Geometry check sheet. Reference: the model listing, model coordinates, mm. Coordinates: 2 decimals unless noted, no trailing zeros. Order: outer loops, then holes, each group sorted by start corner. A loop starts at its lowest first (then second) coordinate and runs counter-clockwise, first axis right, second up. Notation, with made-up numbers: (-34.75, 63) - (-20.75, 63) arc R31 ccw to (-20.75, 96) - close; hole circle Ø7 at (-2, 40). An arc over 180 degrees is marked (long way). Use CSV: the item, a comma, the result in double quotes. Start each with the question number.
1) Sectioned sample at A-A, the plane x = 106.5. Record the cut outline in (y, z), and give its area (3 significant figures).
2) Depth check by flat-ended pin: P1, Ø5, axis at x = 450, z = 0, coming from the +Y side; P2, Ø3.5, axis at x = 153.5, y = 9, coming from the -Z side. Enter the tip coordinate at first touch or a pass-through.
3) Thickness scan on probe 1 along Z at (x, y) = (210, 12.35); probe 2 along Z at (x, y) = (570, 5.75); probe 3 along Z at (x, y) = (63.5, 6.5). Record the ranges inside material, lowest first. Write a range as [from, to].
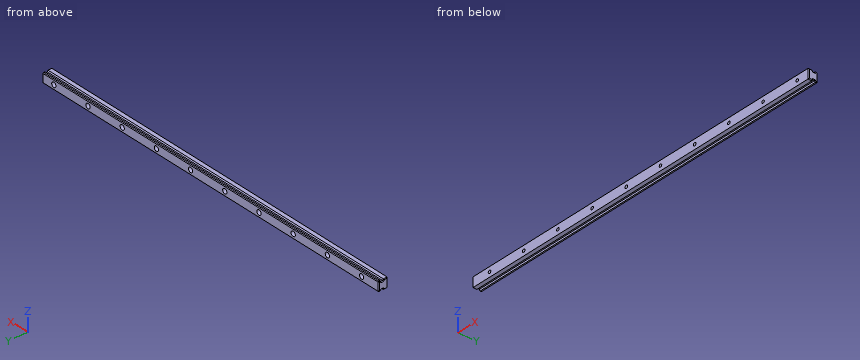
from build123d import *

# Parameters (mm, degrees)
BOSS_EXTRUDE1_DEPTH = 590
CHAMFER1_SIZE       = 1
CHAMFER2_SIZE       = 1
SKETCH2_R           = 3.75
CUT_EXTRUDE1_DEPTH  = 5.3
SKETCH3_R           = 2.25
CUT_EXTRUDE2_DEPTH  = 591.111802966
LPATTERN1_COUNT     = 67
LPATTERN1_PITCH     = 60


with BuildPart() as part:
    # Sketch1 → Boss-Extrude1 (new body)
    with BuildSketch(Plane(origin=(0, 0, 0), x_dir=(0, 0, -1), z_dir=(1, 0, 0))):
        Polygon((-7.5, 0), (7.5, 0), (7.5, 6), (5.5, 7), (5.5, 10), (7.5, 11), (7.5, 13), (6.5, 14), (-6.5, 14), (-7.5, 13), (-7.5, 11), (-5.5, 10), (-5.5, 7), (-7.5, 6), align=None)
    extrude(amount=BOSS_EXTRUDE1_DEPTH)

    # Chamfer1
    chamfer1_edges = [part.edges().sort_by_distance(p)[0] for p in [
        (0, 6.5, 6.5),
        (0, 8.5, 5.5),
        (0, 10.5, 6.5),
        (0, 12, 7.5),
        (0, 13.5, 7),
        (0, 14, 0),
        (0, 13.5, -7),
        (0, 12, -7.5),
        (0, 10.5, -6.5),
        (0, 8.5, -5.5),
        (0, 6.5, -6.5),
        (0, 3, -7.5),
        (0, 0, 0),
        (0, 3, 7.5),
    ]]
    chamfer(chamfer1_edges, length=CHAMFER1_SIZE)

    # Chamfer2
    chamfer2_edges = [part.edges().sort_by_distance(p)[0] for p in [
        (590, 3, -7.5),
        (590, 6.5, -6.5),
        (590, 8.5, -5.5),
        (590, 10.5, -6.5),
        (590, 12, -7.5),
        (590, 13.5, -7),
        (590, 14, 0),
        (590, 13.5, 7),
        (590, 12, 7.5),
        (590, 10.5, 6.5),
        (590, 3, 7.5),
        (590, 8.5, 5.5),
        (590, 6.5, 6.5),
        (590, 0, 0),
    ]]
    chamfer(chamfer2_edges, length=CHAMFER2_SIZE)

    # Sketch2 → Cut-Extrude1 (cut)
    with BuildSketch(Plane(origin=(0, 14, 0), x_dir=(1, 0, 0), z_dir=(0, 1, 0))):
        with Locations(Location((570, 0, 0), (0, 0, 270))):
            Circle(SKETCH2_R)
    cut_extrude1 = extrude(amount=-CUT_EXTRUDE1_DEPTH, mode=Mode.SUBTRACT)

    # Sketch3 → Cut-Extrude2 (cut, through all)
    with BuildSketch(Plane(origin=(0, 8.7, 0), x_dir=(1, 0, 0), z_dir=(0, 1, 0))):
        with Locations(Location((570, 0, 0), (0, 0, 270))):
            Circle(SKETCH3_R)
    cut_extrude2 = extrude(amount=-CUT_EXTRUDE2_DEPTH, mode=Mode.SUBTRACT)

    # LPattern1: Cut-Extrude1, Cut-Extrude2 ×67
    with Locations(*[(-i * LPATTERN1_PITCH, 0, 0) for i in range(1, LPATTERN1_COUNT)]):
        add(cut_extrude1, mode=Mode.SUBTRACT)
        add(cut_extrude2, mode=Mode.SUBTRACT)


solid = part.part
Evaluation:
1,outline,"(0, -7.5) - (6, -7.5) - (7, -5.5) - (10, -5.5) - (11, -7.5) - (13, -7.5) - (14, -6.5) - (14, 6.5) - (13, 7.5) - (11, 7.5) - (10, 5.5) - (7, 5.5) - (6, 7.5) - (0, 7.5) - close"
1,area,"193 mm²"
2,P1,"y = 8.7"
2,P2,"z = -7"
3,probe 1,"[-7.5, -3.75], [3.75, 7.5]"
3,probe 2,"[-7.5, -2.25], [2.25, 7.5]"
3,probe 3,"[-6.5, 6.5]"
